Check sheet for the modelled part. Datum: model origin and axes. Units: mm. Round coordinates to 2 decimals unless told otherwise and drop trailing zeros. Write each loop counter-clockwise with the first axis right and the second up, starting at its lowest first coordinate (ties: lowest second). Pieces come first, ordered by that corner, then holes. Notation, with made-up numbers: M 72,-31.5 L 126,-31.5 A9 cw 126,-26.5 Z; hole C 75,16.5 d4. An arc over 180 degrees is marked long. Put each result on its own line as item: value.
```python
from build123d import *

# Parameters (mm, degrees)
BOSS_EXTRU_2_DEPTH      = 31.242
ESQUISSE1_6_W           = 205.926380568
ESQUISSE1_6_H           = 152.99378218
ENL_V_MAT_EXTRU_3_DEPTH = 1
CONG_2_R                = 1


with BuildPart() as part:
    # Esquisse1 → Boss.-Extru.2 (new body)
    with BuildSketch(Plane.XY):
        with BuildLine():
            Line((-102.649, -83.693), (102.649, -83.693))
            ThreePointArc((102.649, -83.693), (109.720067812, -80.764067812), (112.649, -73.693))
            Line((112.649, -73.693), (112.649, 73.693))
            ThreePointArc((112.649, 73.693), (109.720067812, 80.764067812), (102.649, 83.693))
            Line((102.649, 83.693), (-102.649, 83.693))
            ThreePointArc((-102.649, 83.693), (-109.720067812, 80.764067812), (-112.649, 73.693))
            Line((-112.649, 73.693), (-112.649, -73.693))
            ThreePointArc((-112.649, -73.693), (-109.720067812, -80.764067812), (-102.649, -83.693))
        make_face()
    extrude(amount=BOSS_EXTRU_2_DEPTH)

    # Esquisse1_6 → Enl_v. mat.-Extru.3 (cut)
    with BuildSketch(Plane.XY):
        Rectangle(ESQUISSE1_6_W, ESQUISSE1_6_H)
    extrude(amount=ENL_V_MAT_EXTRU_3_DEPTH, mode=Mode.SUBTRACT)

    # Cong_2
    cong_2_edges = [part.edges().sort_by_distance(p)[0] for p in [
        (112.649, 0, 0),
        (109.720067812, 80.764067812, 0),
        (0, 83.693, 0),
        (-109.720067812, 80.764067812, 0),
        (-112.649, 0, 0),
        (-109.720067812, -80.764067812, 0),
        (0, -83.693, 0),
        (109.720067812, -80.764067812, 0),
    ]]
    fillet(cong_2_edges, radius=CONG_2_R)


solid = part.part
```
1. Depth check by flat-ended pin: pin 1 Ø5 at (x, y) = (-33.5, 34) entering from -Z; pin 2 Ø0.5 at (y, z) = (19.5, 0.5) entering from +X; pin 3 Ø0.5 at (x, z) = (15.5, 0.5) entering from +Y. Enter the tip coordinate at first touch or a pass-through.
Computed values:
pin 1: stops at z = 1
pin 2: stops at x = 112.62
pin 3: stops at y = 83.66
2. Release check for a two-part mould opening along Y. For faces 1 (the flat face through (-1, 1, 1)), 2 (the cylindrical face through (109.797, 80.686, 15.909)), 3 (the cylindrical face through (109.642, -80.841, 15.909)) record: +Y half, -Y half, draft (parallel to the pull), parting line (faces both ways), or undercut.
Computed values:
face 1: undercut
face 2: +Y half
face 3: -Y half
3. Cross-section at A-A (y = 41.5). Enter the section's corners in (x, z), then the cut area to 3 significant figures.
Computed values:
outline: M -112.65,1 A1 ccw -111.65,0 L -102.96,0 L -102.96,1 L 102.96,1 L 102.96,0 L 111.65,0 A1 ccw 112.65,1 L 112.65,31.24 L -112.65,31.24 Z
area: 6,830 mm2
4. Cross-section at B-B (x = 98.5). Enter the section's corners in (y, z), then the cut area to 3 significant figures.
Computed values:
outline: M -83.69,1 A1 ccw -82.69,0 L -76.5,0 L -76.5,1 L 76.5,1 L 76.5,0 L 82.69,0 A1 ccw 83.69,1 L 83.69,31.24 L -83.69,31.24 Z
area: 5,080 mm2
5. Scan lines: probe 1 along Z at (x, y) = (-90.5, 37); probe 2 along Y at (x, z) = (103, 3). Record each from-to range of solid material in increasing order.
Computed values:
probe 1: z = 1 to 31.24
probe 2: y = -83.69 to 83.69
